from build123d import *

# Parameters (mm, degrees)
F1_DEPTH = 25.4
F2_W     = 12.7
F2_H     = 19.05
F3_DEPTH = 38.099740899
F4_W     = 38.1
F4_H     = 12.7
F5_DEPTH = 2.54
F7_DEPTH = 12.701
F9_DEPTH = 12.3912550856


with BuildPart() as f1:
    # F0 (on Front) → F1 (new body)
    with BuildSketch(Plane.XZ):
        Polygon((-31.4954862574, 31.774422986), (-31.4954862574, 0.024422986), (6.6032546415, 0.024422986), (6.6032546415, 31.4646780716), align=None)
    extrude(amount=F1_DEPTH)

    # F2 (on face) → F3 (cut, through all)
    with BuildSketch(Plane.YZ.offset(6.6032546415)):
        with Locations((-19.05, 21.9396780716)):
            Rectangle(F2_W, F2_H)
    extrude(amount=-F3_DEPTH, mode=Mode.SUBTRACT)

    # F4 (on face) → F5 (cut)
    with BuildSketch(Plane(origin=(0.2562291336, 0, 31.5162797473), x_dir=(0.9999669527, 0, -0.0081297878), z_dir=(0.0081297878, 0, 0.9999669527))):
        with Locations((-12.7027647333, -19.05)):
            Rectangle(F4_W, F4_H)
    extrude(amount=-F5_DEPTH, mode=Mode.SUBTRACT)

    # F6 (on face) → F7 (cut, through all)
    with BuildSketch(Plane.XZ.offset(12.7)):
        Polygon((-6.0963256581, 31.5679263764), (6.6032546415, 12.4146780716), (6.6032546415, 31.4646780716), align=None)
    extrude(amount=-F7_DEPTH, mode=Mode.SUBTRACT)

    # F8 (on face) → F9 (cut, through all)
    with BuildSketch(Plane.XY.offset(12.4146780716)):
        Polygon((6.6032546415, -25.4), (6.6032546415, -12.7), (-5.669398699, -25.4), align=None)
    extrude(amount=-F9_DEPTH, mode=Mode.SUBTRACT)


solid = f1.part
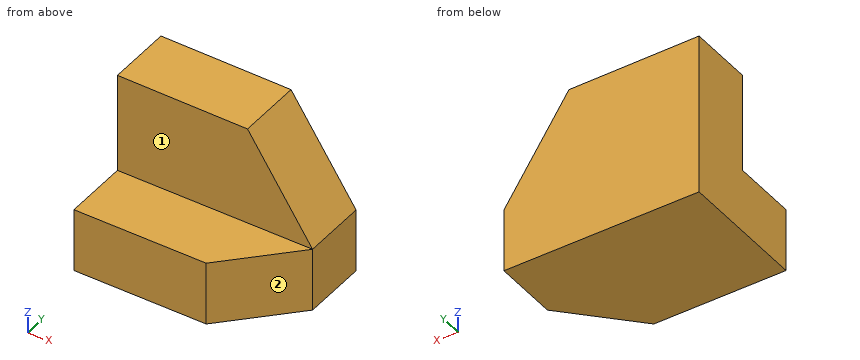
The model under review builds one solid part; all positions refer to its coordinate system, in mm. Face numbers are marked on the shaded views. A direction names the side the tool comes from. Give positions to 0.01 mm unless a question says otherwise; leave off trailing zeros. Order: outer loops, then holes, each group sorted by start corner. A loop starts at its lowest first (then second) coordinate and runs counter-clockwise, first axis right, second up. Notation, with made-up numbers: M -13,-3 L 22,-3 A16 ccw 22,25 Z; hole C 58.5,76.5 d9. An arc over 180 degrees is marked long. Use one line per item in the form item = value. Start each with the question number.
Item 1: To check wall thickness, follow line 1 along Y through (x, z) = (-17, 14.5); line 2 along Z through (x, y) = (-28, -23.25); line 3 along Z through (x, y) = (-7.5, -3.5). State the ranges of each line that lie inside material, in increasing order. Write a range as from..to.
Item 2: Insertion check: pin 1 Ø8 at (x, y) = (-17, -7.5) entering from +Z; pin 2 Ø1.5 at (x, z) = (-20, 18.5) entering from -Y; pin 3 Ø6.5 at (x, y) = (-15, -20.5) entering from +Z; pin 4 Ø1 at (y, z) = (-18, 13.5) entering from -X. Each pin has a flat end and moves straight along its axis. Give the tip position at first contact, or say it passes through.
Item 3: We need section A-A on y = -10. Give the boundary of the cut face in (x, z), plus the area to 3 significant figures.
Item 4: We need section B-B on x = -28.5. Give the boundary of the cut face in (y, z).
Item 5: We need section D-D on x = -21.5. Give the boundary of the cut face in (y, z).
Item 6: For the marked faces 1 and 2, list the 3-axis set-ups (+Z, -Z, +X, -X, +Y, -Y) from which the entire face can be reached by the end or side of a thin tool; tool diameter is ignored.
Item 7: We need section C-C on z = 13. Give the boundary of the cut face in (x, y).
Completed:
q1.line_1 = -12.7..0
q1.line_2 = 0.02..12.41
q1.line_3 = 0.02..31.58
q2.pin_1 = 31.69
q2.pin_2 = -12.7
q2.pin_3 = 12.41
q2.pin_4 = through
q3.outline = M -31.5,0.02 L 6.6,0.02 L 6.6,12.41 L -6.1,31.57 L -31.5,31.77 Z
q3.area = 1,080 mm²
q4.outline = M -25.4,0.02 L 0,0.02 L 0,31.75 L -12.7,31.75 L -12.7,12.41 L -25.4,12.41 Z
q5.outline = M -25.4,0.02 L 0,0.02 L 0,31.69 L -12.7,31.69 L -12.7,12.41 L -25.4,12.41 Z
q6.face_1 = +Z, +X, -X, -Y
q6.face_2 = +Z, -Z, +X, -Y
q7.outline = M -31.5,-12.7 L 6.22,-12.7 L 6.22,0 L -31.5,0 Z
